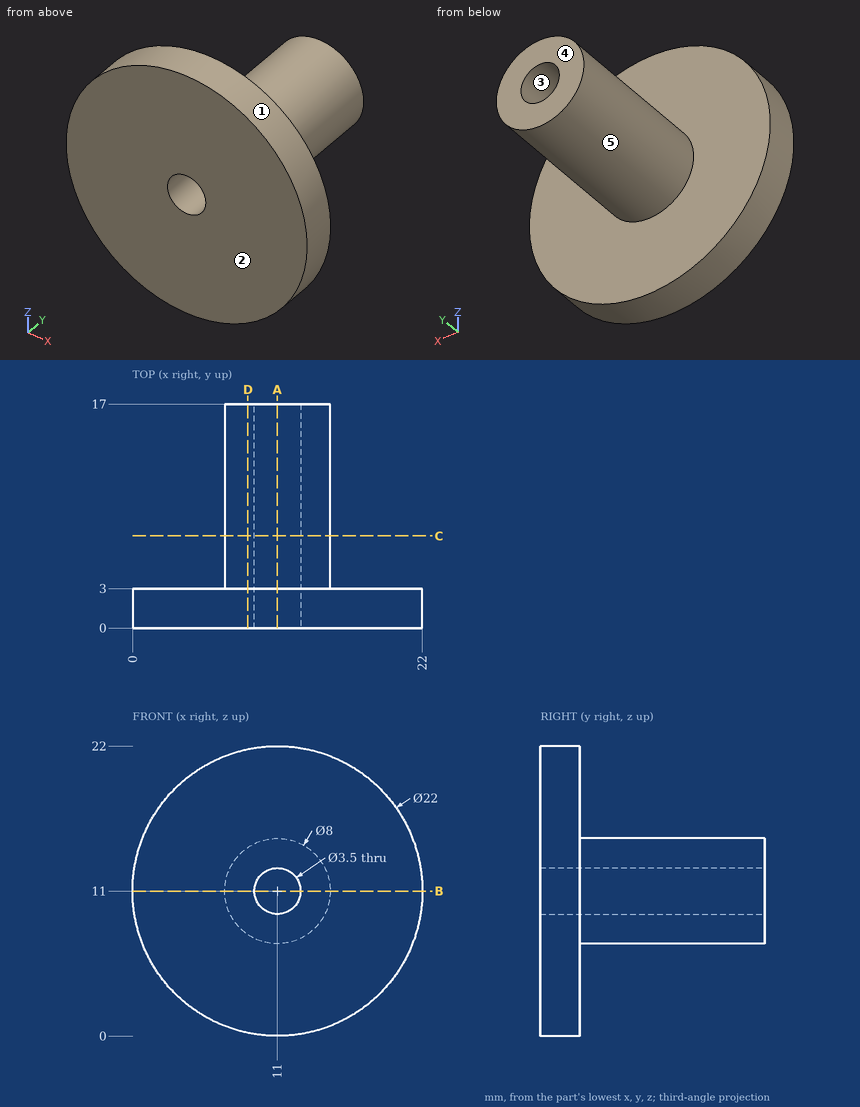
Here's the drawing with two shaded views (mm, measured from the low corner). I have some questions. A direction names the side the tool comes from. Coordinates: 2 decimals unless noted, no trailing zeros. Write each loop counter-clockwise with the first axis right and the second up, starting at its lowest first coordinate (ties: lowest second). Pieces come first, ordered by that corner, then holes. Notation, with made-up numbers: (38, -15.75) -> (82, -15.75) arc R29 cw to (82, 19.25) -> close; hole circle Ø10 at (-20.5, 82.25). An arc over 180 degrees is marked (long way). Use a Markdown table: item, result. Add a question column.
(1) If we section it at B-B, the plane z = 11: Write out the boundary of the cut face in (x, y).
(2) If we section it at A-A, the plane x = 11: Write out the boundary of the cut face in (y, z).
(3) For the marked faces 4 and 5, which set-ups out of +Z, -Z, +X, -X, +Y, -Y let a thin tool reach every point of the face, with its end or its side?
(4) We'd pull the mould along Z, two halves only. Please class the marked faces 1, 2 and 3: +Z half, -Z half, draft (parallel to the pull), parting line (faces both ways), or undercut.
(5) Please list where these lines run through material, in increasing order: line 1 (Z direction, x = 11, y = 7.5); line 2 (X direction, y = 2.5, z = 11).
(6) I'm going to push flat-ended pins straight in: P1, Ø10, axis at y = 6.5, z = 3, coming from the -X side; P2, Ø1, axis at y = 7.5, z = 7.5, coming from the +X side; P3, Ø3, axis at x = 11, y = 6.5, coming from the -Z side. Where does each tip first touch, or does it pass through?
(7) If we section it at D-D, the plane x = 8.75: Write out the boundary of the cut face in (y, z), and give its area (3 significant figures).
(8) If we section it at C-C, the plane y = 7: Write out the boundary of the cut face in (x, z).
Outcome:
| question | item | result |
|---|---|---|
| 1 | outline | (0, 0) -> (9.25, 0) -> (9.25, 17) -> (7, 17) -> (7, 3) -> (0, 3) -> close; (12.75, 0) -> (22, 0) -> (22, 3) -> (15, 3) -> (15, 17) -> (12.75, 17) -> close |
| 2 | outline | (0, 0) -> (3, 0) -> (3, 7) -> (17, 7) -> (17, 9.25) -> (0, 9.25) -> close; (0, 12.75) -> (17, 12.75) -> (17, 15) -> (3, 15) -> (3, 22) -> (0, 22) -> close |
| 3 | face 4 | +Z, -Z, +X, -X, +Y |
| 3 | face 5 | +Y |
| 4 | face 1 | parting line |
| 4 | face 2 | draft |
| 4 | face 3 | undercut |
| 5 | line 1 | z = 7 to 9.25, 12.75 to 15 |
| 5 | line 2 | x = 0 to 9.25, 12.75 to 22 |
| 6 | P1 | stops at x = 0.93 |
| 6 | P2 | stops at x = 13.65 |
| 6 | P3 | stops at z = 7 |
| 7 | outline | (0, 0.23) -> (3, 0.23) -> (3, 7.69) -> (17, 7.69) -> (17, 14.31) -> (3, 14.31) -> (3, 21.77) -> (0, 21.77) -> close |
| 7 | area | 157 mm^2 |
| 8 | outline | circle Ø8 at (11, 11); hole circle Ø3.5 at (11, 11) |
